```python
from build123d import *

# Parameters (mm, degrees)
F0_W     = 76.2
F0_H     = 101.6
F0_R     = 3.2639
F1_DEPTH = 19.05
F2_R     = 2.5527
F3_DEPTH = 19.05
F4_SIZE  = 0.508


with BuildPart() as f1:
    # F0 (on Front) → F1 (new body)
    with BuildSketch(Plane.XZ):
        Rectangle(F0_W, F0_H)
        with Locations((-19.05, -25.4)):
            Circle(F0_R, mode=Mode.SUBTRACT)
        with Locations((19.05, -25.4)):
            Circle(F0_R, mode=Mode.SUBTRACT)
        with Locations((-19.05, 25.4)):
            Circle(F0_R, mode=Mode.SUBTRACT)
        with Locations((19.05, 25.4)):
            Circle(F0_R, mode=Mode.SUBTRACT)
    extrude(amount=F1_DEPTH)

    # F2 (on face) → F3 (cut)
    with BuildSketch(Plane(origin=(0, 0, -50.8), x_dir=(1, 0, 0), z_dir=(0, 0, -1))):
        with Locations((-19.05, 9.525)):
            Circle(F2_R)
        with Locations((19.05, 9.525)):
            Circle(F2_R)
    extrude(amount=-F3_DEPTH, mode=Mode.SUBTRACT)

    # F4
    f4_edges = [f1.edges().sort_by_distance(p)[0] for p in [
        (38.1, -19.05, 0),
        (0, -19.05, 50.8),
        (-38.1, -19.05, 0),
        (0, -19.05, -50.8),
        (-22.3139, -19.05, -25.4),
        (15.7861, -19.05, -25.4),
        (-22.3139, -19.05, 25.4),
        (15.7861, -19.05, 25.4),
        (-38.1, -9.525, 50.8),
        (-38.1, -9.525, -50.8),
        (-38.1, 0, 0),
        (0, 0, -50.8),
        (38.1, -9.525, -50.8),
        (-21.6027, -9.525, -50.8),
        (16.4973, -9.525, -50.8),
        (38.1, 0, 0),
        (0, 0, 50.8),
        (-22.3139, 0, -25.4),
        (15.7861, 0, -25.4),
        (-22.3139, 0, 25.4),
        (15.7861, 0, 25.4),
        (38.1, -9.525, 50.8),
    ]]
    chamfer(f4_edges, length=F4_SIZE)


solid = f1.part
```
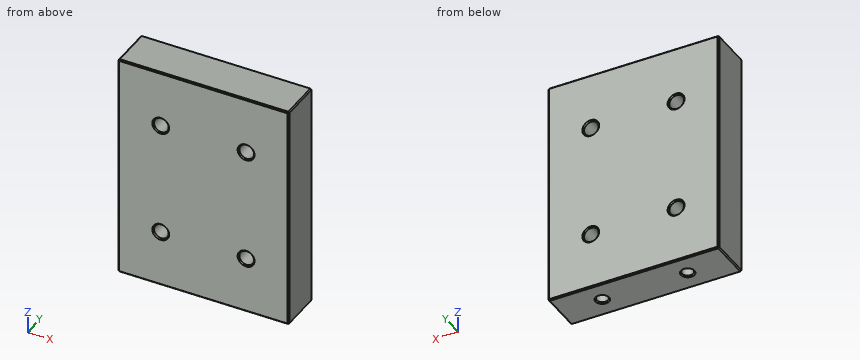
Can you work these out from the model? Positions are in its coordinate system, mm. Give positions to 0.01 mm unless a question says otherwise; leave off trailing zeros. Write each loop counter-clockwise with the first axis right and the second up, starting at its lowest first coordinate (ties: lowest second). Pieces come first, ordered by that corner, then holes. Notation, with made-up numbers: (88.25, -8) -> (140.25, -8) arc R23 ccw to (140.25, 9) -> close; hole circle Ø8 at (86.25, -26). An arc over 180 degrees is marked (long way). Write item = value, one per line.
(1) Suppose I cut it at A-A on z = -25.4. Write out the boundary of the cut face in (x, y).
Worked out:
outline = (-38.1, -18.54) -> (-37.59, -19.05) -> (-22.82, -19.05) -> (-22.31, -18.54) -> (-22.31, -0.51) -> (-22.82, 0) -> (-37.59, 0) -> (-38.1, -0.51) -> close; (-15.79, -18.54) -> (-15.28, -19.05) -> (15.28, -19.05) -> (15.79, -18.54) -> (15.79, -0.51) -> (15.28, 0) -> (-15.28, 0) -> (-15.79, -0.51) -> close; (22.31, -18.54) -> (22.82, -19.05) -> (37.59, -19.05) -> (38.1, -18.54) -> (38.1, -0.51) -> (37.59, 0) -> (22.82, 0) -> (22.31, -0.51) -> close
(2) Suppose I cut it at C-C on y = -15.5. Write out the boundary of the cut face in (x, z), then the cut area to 3 significant figures.
Worked out:
outline = (-38.1, -50.29) -> (-37.59, -50.8) -> (37.59, -50.8) -> (38.1, -50.29) -> (38.1, 50.29) -> (37.59, 50.8) -> (-37.59, 50.8) -> (-38.1, 50.29) -> close; hole circle Ø6.53 at (-19.05, -25.4); hole circle Ø6.53 at (-19.05, 25.4); hole circle Ø6.53 at (19.05, -25.4); hole circle Ø6.53 at (19.05, 25.4)
area = 7,610 mm^2
(3) I'm going to push flat-ended pins straight in: P1, Ø8.5, axis at x = 19.05, z = -25.4, coming from the +Y side; P2, Ø1.5, axis at x = 20, y = -10, coming from the -Z side. Where does each tip first touch, or does it pass through?
Worked out:
P1 = 0
P2 = -31.75
(4) I need wall thicknesses on probe 1 along Z at (x, y) = (19.05, -12); probe 2 along Z at (x, y) = (19.05, -5.5); probe 3 along Y at (x, z) = (-19.05, -37.75). Which ranges of each line are inside material? Lowest first, please. Write a range as from..to.
Worked out:
probe_1 = -31.75..-28.66, -22.14..22.14, 28.66..50.8
probe_2 = -50.8..-28.66, -22.14..22.14, 28.66..50.8
probe_3 = -19.05..-12.08, -6.97..0
(5) Suppose I cut it at B-B on x = 19.05. Count the separate pieces of the cut face and the enclosed holes in it, then the cut area to 3 significant figures.
Worked out:
separate_pieces = 3
enclosed_holes = 0
area = 1,590 mm^2
